from build123d import *

# Parameters (mm, degrees)
F0_W     = 15
F0_H     = 10
F0_R     = 2.5
F1_DEPTH = 5
F3_DEPTH = 31
F4_R     = 4.5
F5_DEPTH = 10
F6_R     = 5


# Not quite as in the source:
# - a feature names something its author has since deleted; it is built from what else it names


with BuildPart() as f1:
    # F0 (on Front) → F1 (new body)
    with BuildSketch(Plane.XZ):
        with Locations((-27.5, 0)):
            Rectangle(F0_W, F0_H)
        Polygon((20, 15), (-20, 15), (-20, 5), (-20, -5), (-20, -15), (20, -15), (20, -5), (20, 5), align=None)
        with Locations((-11, 0)):
            Circle(F0_R, mode=Mode.SUBTRACT)
        with Locations((11, 0)):
            Circle(F0_R, mode=Mode.SUBTRACT)
        with Locations((27.5, 0)):
            Rectangle(F0_W, F0_H)
    extrude(amount=F1_DEPTH)

    # F2 (on face) → F3 (cut)
    with BuildSketch(Plane(origin=(0, 0, -15), x_dir=(1, 0, 0), z_dir=(0, 0, -1))):
        with BuildLine():
            ThreePointArc((-1.5, 5), (0, 3.5), (1.5, 5))
            Line((1.5, 5), (-1.5, 5))
        make_face()
    extrude(amount=-F3_DEPTH, mode=Mode.SUBTRACT)

    # F4 (on face) → F5 (join)
    with BuildSketch(Plane(origin=(0, 0, 0), x_dir=(-1, 0, 0), z_dir=(0, 1, 0))):
        with BuildLine():
            ThreePointArc((50, 0), (42.588190451, 9.6592582629), (31.3397459622, 5))
            Line((31.3397459622, 5), (35, 5))
            Line((35, 5), (35, -5))
            Line((35, -5), (31.3397459622, -5))
            ThreePointArc((31.3397459622, -5), (42.588190451, -9.6592582629), (50, 0))
        make_face()
        with Locations((40, 0)):
            Circle(F4_R, mode=Mode.SUBTRACT)
        with BuildLine():
            Line((-35, 5), (-31.3397459622, 5))
            ThreePointArc((-31.3397459622, 5), (-50, 0), (-31.3397459622, -5))
            Line((-31.3397459622, -5), (-35, -5))
            Line((-35, -5), (-35, 5))
        make_face()
        with Locations((-40, 0)):
            Circle(F4_R, mode=Mode.SUBTRACT)
        with BuildLine():
            ThreePointArc((-31.3397459622, -5), (-30.3407417371, -2.588190451), (-30, 0))
            ThreePointArc((-30, 0), (-30.3407417371, 2.588190451), (-31.3397459622, 5))
            Line((-31.3397459622, 5), (-35, 5))
            Line((-35, 5), (-35, -5))
            Line((-35, -5), (-31.3397459622, -5))
        make_face()
        with BuildLine():
            Line((35, 5), (31.3397459622, 5))
            ThreePointArc((31.3397459622, 5), (30, 0), (31.3397459622, -5))
            Line((31.3397459622, -5), (35, -5))
            Line((35, -5), (35, 5))
        make_face()
    extrude(amount=-F5_DEPTH)

    # F6
    f6_edges = [f1.edges().sort_by_distance(p)[0] for p in [
        (20, -2.5, -15),
        (20, -2.5, 15),
        (-20, -2.5, 15),
        (-20, -2.5, -15),
    ]]
    fillet(f6_edges, radius=F6_R)


solid = f1.part
Here's how the part is built. I have some questions about the finished solid (model axes, mm). A direction names the side the tool comes from. Coordinates: 2 decimals unless noted, no trailing zeros. Write each loop counter-clockwise with the first axis right and the second up, starting at its lowest first coordinate (ties: lowest second). Pieces come first, ordered by that corner, then holes.
Item 1: I want a section at A-A on y = -8.25. Write out the boundary of the cut face in (x, z), and give its area (3 significant figures).
Item 2: On a 3-axis mill with a long thin cutter (end or side, diameter ignored), from which of +Z, -Z, +X, -X, +Y, -Y can I reach the whole of each face in a straight line? I mean faces 1 (the cylindrical face through (0, -3.5, -0.2)), 2 (the flat face through (26, -2, -5)), 3 (the flat face through (-20, -2, 8)). Say none if no direction works.
Item 3: I want a section at C-C on y = -2.25. Write out the boundary of the cut face in (x, z), and give its area (3 significant figures).
Item 4: If we mould it in two halves opening along Z, with no side actions, what happens to faces 4 (the cylindrical face through (35.708, -4.93, 1.352)), 5 (the cylindrical face through (8.5, -2.5, 0.1)), 6 (the cylindrical face through (-19, -3, 13)), 7 (the cylindrical face through (-19, -3, -13))? For each: +Z half, -Z half, draft (parallel to the pull), parting line (faces both ways), or undercut.
Item 5: Will these pins go through, and if not, where does the flat tip stop? pin 1 (1.5 mm diameter, centred on y = -3.5, z = 8.5, fed in from -X); pin 2 (2 mm diameter, centred on x = -35.5, y = -7.5, fed in from +Z); pin 3 (2.5 mm diameter, centred on y = -3.5, z = -7.5, fed in from +X); pin 4 (10.5 mm diameter, centred on x = -40, z = 0, fed in from +Y).
Item 6: I want a section at B-B on x = 40. Write out the boundary of the cut face in (y, z), and give its area (3 significant figures).
Item 7: If I drill on line 1 (X direction, y = -3.75, z = 7.25); line 2 (X direction, y = -5.75, z = 1); line 3 (Z direction, x = 11, y = -1.7), over which ranges is the centre line in solid material (lowest first)?
Item 8: I want a section at D-D on x = -11. Write out the boundary of the cut face in (y, z), and give its area (3 significant figures).
Findings below:
1. outline: circle Ø20 at (-40, 0); circle Ø20 at (40, 0); hole circle Ø9 at (-40, 0); hole circle Ø9 at (40, 0)
1. area: 501 mm2
2. face 1: +Z, -Z, -Y
2. face 2: -Z, +Y, -Y
2. face 3: +Z, +Y, -Y
3. outline: (-31.34, -5) - (-20, -5) - (-20, -10) arc R5 ccw to (-15, -15) - (15, -15) arc R5 ccw to (20, -10) - (20, -5) - (31.34, -5) arc R10 ccw (long way) to (31.34, 5) - (20, 5) - (20, 10) arc R5 ccw to (15, 15) - (-15, 15) arc R5 ccw to (-20, 10) - (-20, 5) - (-31.34, 5) arc R10 ccw (long way) to start; hole circle Ø9 at (-40, 0); hole circle Ø5 at (-11, 0); hole circle Ø5 at (11, 0); hole circle Ø9 at (40, 0)
3. area: 1,850 mm2
4. face 4: undercut
4. face 5: undercut
4. face 6: +Z half
4. face 7: -Z half
5. pin 1: stops at x = -46.32
5. pin 2: stops at z = 9.37
5. pin 3: stops at x = 47.81
5. pin 4: stops at y = 0
6. outline: (-10, -10) - (0, -10) - (0, -4.5) - (-10, -4.5) - close; (-10, 4.5) - (0, 4.5) - (0, 10) - (-10, 10) - close
6. area: 110 mm2
7. line 1: x = -46.89 to -33.11, -20 to -0.83, 0.83 to 20, 33.11 to 46.89
7. line 2: x = -49.95 to -44.39, -35.61 to -30.05, 30.05 to 35.61, 44.39 to 49.95
7. line 3: z = -15 to -2.5, 2.5 to 15
8. outline: (-5, -15) - (0, -15) - (0, -2.5) - (-5, -2.5) - close; (-5, 2.5) - (0, 2.5) - (0, 15) - (-5, 15) - close
8. area: 125 mm2
